Geometry: final body of the model. Coordinates: model frame, mm. A direction names the side the tool comes from. Coordinates: 2 decimals unless noted, no trailing zeros. Order: outer loops, then holes, each group sorted by start corner. A loop starts at its lowest first (then second) coordinate and runs counter-clockwise, first axis right, second up. Notation, with made-up numbers: (-18, -15.5) -> (2, -15.5) arc R19 cw to (2, 1.5) -> close; hole circle Ø3 at (75.5, -27). An arc over 180 degrees is marked (long way). Answer in a Markdown table with one row per item. Add a question column.
1) Ray query, line 1 (X direction, y = 1, z = 0.7); line 2 (Y direction, x = 0, z = 1.8); line 3 (Y direction, x = 1.5, z = 1.05). Return the intervals inside material, ascending. Write a range as from..to.
2) Section query C-C on y = 0.25. Count the separate pieces of the cut face and the enclosed holes in it, then the cut area to 3 significant figures.
3) Set-up query: faces 1 (the face through (-1, 5, 2.5)), 2 (the face through (-0.899, -4.047, 1.754)). Return all of +Z, -Z, +X, -X, +Y, -Y with unobstructed straight access to the full face (end or side cutting, diameter ignored); none if empty.
4) Contact query for flat-ended pins moving along their axis: P1, Ø1, axis at x = -1.5, z = 0.5, coming from the -Y side; P2, Ø2, axis at x = 1.94, y = 0.63, coming from the +Z side; P3, Ø1.5, axis at y = 1.5, z = 1.5, coming from the +X side. Output: stop coordinate, or through.
5) Section query A-A on x = 0. Return the cut outline in (y, z), then the cut area to 3 significant figures.
Autodesk Inventor part; units mm, degrees
ref_plane "YZ Plane" through (0, 0, 0) normal (1, 0, 0) x (0, 1, 0)
ref_plane "XZ Plane" through (0, 0, 0) normal (0, 1, 0) x (-1, 0, 0)
ref_plane "XY Plane" through (0, 0, 0) normal (0, 0, 1) x (1, 0, 0)
sketch "Sketch1" plane through (0, 0, 0) normal (0, 0, 1) x (1, 0, 0)
  circle A0 centre (0, 0) radius 6
  dimension "d0" = 12
extrude "Extrusion1" add sketch "Sketch1" along normal blind 2.5
fillet "Fillet1" radius 0.5 2 edges at (-6, 0, 2.5) (-6, 0, 0)
sketch "Sketch2" plane through (0, 0, 2.5) normal (0, 0, 1) x (1, 0, 0)
  circle A0 centre (0, 0) radius 4.1457
extrude "Extrusion2" cut sketch "Sketch2" against normal blind 1
fillet "Fillet2" radius 0.5 1 edges at (-4.1457, 0, 2.5)
sketch "Sketch3" plane through (0, 0, 1.5) normal (0, 0, 1) x (1, 0, 0)
  circle A0 centre (0, 0) radius 0.5
  dimension "d7" = 1
extrude "Extrusion3" cut sketch "Sketch3" against normal through all
sketch "Sketch4" plane through (0, 0, 1.5) normal (0, 0, 1) x (1, 0, 0)
  circle A0 centre (0, 2.0358) radius 0.9294
  point P0 (0, 0)
extrude "Extrusion4" cut sketch "Sketch4" against normal blind 1.5
pattern_circular "Circular Pattern1" count 5 over 360 about axis through (0, 0, 1.5) along (0, 0, -1) of "Extrusion2", "Extrusion4"
properties part number "Wheel IT_CPY"
Result:
| question | item | result |
|---|---|---|
| 1 | line 1 | -5.92..-2.79, -1.08..1.08, 2.79..5.92 |
| 1 | line 2 | -6..-4.15, 4.15..6 |
| 1 | line 3 | -5.81..-2.53, -0.77..-0.19, 1.45..5.81 |
| 2 | separate pieces | 4 |
| 2 | enclosed holes | 0 |
| 2 | area | 15.0 mm2 |
| 3 | face 1 | +Z, +X, -X, +Y, -Y |
| 3 | face 2 | +Z |
| 4 | P1 | y = -5.92 |
| 4 | P2 | z = 1.5 |
| 4 | P3 | x = 5.95 |
| 5 | outline | (-6, 0.5) arc R0.5 ccw to (-5.5, 0) -> (-0.5, 0) -> (-0.5, 1.5) -> (-4.15, 1.5) -> (-4.15, 2) arc R0.5 ccw to (-4.65, 2.5) -> (-5.5, 2.5) arc R0.5 ccw to (-6, 2) -> close; (0.5, 0) -> (1.11, 0) -> (1.11, 1.5) -> (0.5, 1.5) -> close; (2.97, 0) -> (5.5, 0) arc R0.5 ccw to (6, 0.5) -> (6, 2) arc R0.5 ccw to (5.5, 2.5) -> (4.65, 2.5) arc R0.5 ccw to (4.15, 2) -> (4.15, 1.5) -> (2.97, 1.5) -> close |
| 5 | area | 17.1 mm2 |
